Geometry: final body of the model. Coordinates: model frame, mm. A direction names the side the tool comes from. Give positions to 0.01 mm unless a question says otherwise; leave off trailing zeros. Write each loop counter-clockwise with the first axis right and the second up, starting at its lowest first coordinate (ties: lowest second). Pieces come first, ordered by that corner, then holes. Notation, with made-up numbers: (25.25, 22) - (51.25, 22) arc R28 cw to (51.25, 41) - close; hole circle Ø7 at (76, -22.75). An arc over 180 degrees is marked (long way). Return JSON: item names as keys, results as strings.
from build123d import *

# Parameters (mm, degrees)
ESQUISSE1_R        = 4.5
BOSS_EXTRU_1_DEPTH = 2.9
ESQUISSE2_W        = 10
ESQUISSE2_H        = 10
BOSS_EXTRU_2_DEPTH = 1.2
ESQUISSE3_W        = 10
ESQUISSE3_H        = 1.2
BOSS_EXTRU_3_DEPTH = 2


with BuildPart() as part:
    # Esquisse1 → Boss.-Extru.1 (new body)
    with BuildSketch(Plane(origin=(0, 0, 0), x_dir=(1, 0, 0), z_dir=(0, 1, 0))):
        with Locations(Location((0, 0, 0), (0, 0, 270))):
            Circle(ESQUISSE1_R)
    extrude(amount=BOSS_EXTRU_1_DEPTH)

    # Esquisse2 → Boss.-Extru.2 (add)
    with BuildSketch(Plane(origin=(0, 2.9, 0), x_dir=(1, 0, 0), z_dir=(0, 1, 0))):
        Rectangle(ESQUISSE2_W, ESQUISSE2_H)
    extrude(amount=BOSS_EXTRU_2_DEPTH)

    # Esquisse3 → Boss.-Extru.3 (add)
    with BuildSketch(Plane(origin=(0, 4.1, 0), x_dir=(1, 0, 0), z_dir=(0, 1, 0))):
        with Locations((0, 4.4)):
            Rectangle(ESQUISSE3_W, ESQUISSE3_H)
        with Locations((0, -4.4)):
            Rectangle(ESQUISSE3_W, ESQUISSE3_H)
    extrude(amount=BOSS_EXTRU_3_DEPTH)


solid = part.part
Q1. Mould query, pull axis Z, two halves, no side actions, for faces 4 (the flat face through (0, 4.1, 0)), 5 (the flat face through (0, 4, 5)), 6 (the cylindrical face through (1.352, 1.43, 4.292)). Classes: pulls with the +Z half, pulls with the -Z half, needs draft (parallel to the pull), parting line crosses it, or undercut.
Answer key:
{"face 4": "undercut", "face 5": "pulls with the +Z half", "face 6": "parting line crosses it"}
Q2. Section query C-C, the plane y = 2.5. Return the cut outline in (x, z).
Answer key:
{"outline": "circle Ø9 at (0, 0)"}
Q3. Section query D-D, the plane x = 1.5. Return the cut outline in (y, z).
Answer key:
{"outline": "(0, -4.24) - (2.9, -4.24) - (2.9, -5) - (6.1, -5) - (6.1, -3.8) - (4.1, -3.8) - (4.1, 3.8) - (6.1, 3.8) - (6.1, 5) - (2.9, 5) - (2.9, 4.24) - (0, 4.24) - close"}
Q4. Pin query (flat end, axial travel): P1, Ø4, axis at x = 1.5, z = 1, coming from the +Y side; P2, Ø1.5, axis at y = 2, z = -1, coming from the -X side; P3, Ø1.5, axis at y = 1, z = -2.5, coming from the -X side. Return the tip coordinate at first contact, or that it passes through.
Answer key:
{"P1": "stops at y = 4.1", "P2": "stops at x = -4.49", "P3": "stops at x = -4.15"}
Q5. Section query B-B, the plane z = 0. Return the cut outline in (x, y).
Answer key:
{"outline": "(-5, 2.9) - (-4.5, 2.9) - (-4.5, 0) - (4.5, 0) - (4.5, 2.9) - (5, 2.9) - (5, 4.1) - (-5, 4.1) - close"}
Q6. Section query A-A, the plane x = 0. Return the cut outline in (y, z).
Answer key:
{"outline": "(0, -4.5) - (2.9, -4.5) - (2.9, -5) - (6.1, -5) - (6.1, -3.8) - (4.1, -3.8) - (4.1, 3.8) - (6.1, 3.8) - (6.1, 5) - (2.9, 5) - (2.9, 4.5) - (0, 4.5) - close"}
Q7. Material intervals for probe 1 along Z at (x, y) = (1.5, 4.25); probe 2 along Y at (x, z) = (-2.5, 0.5); probe 3 along Y at (x, z) = (4.5, -1.5), sorted ascending. Write a range as [from, to].
Answer key:
{"probe 1": "z = [-5, -3.8], [3.8, 5]", "probe 2": "y = [0, 4.1]", "probe 3": "y = [2.9, 4.1]"}
Q8. Set-up query: faces 1 (the flat face through (5, 3.8, 0.1)), 2 (the flat face through (-1.2, 2.9, -4.5)), 3 (the flat face through (0, 5, 3.8)). Return all of +Z, -Z, +X, -X, +Y, -Y with unobstructed straight access to the full face (end or side cutting, diameter ignored); none if empty.
Answer key:
{"face 1": "+Z, -Z, +X, +Y, -Y", "face 2": "-Y", "face 3": "+X, -X, +Y"}
